Can you work these out from the model? Positions are in its coordinate system, mm. A direction names the side the tool comes from. Coordinates: 2 decimals unless noted, no trailing zeros. Order: outer loops, then holes, each group sorted by start corner. A loop starts at its lowest first (then second) coordinate and runs counter-clockwise, first axis right, second up. Notation, with made-up numbers: (77.5, 77) -> (110.5, 77) arc R19 cw to (110.5, 112) -> close; hole circle Ø1 at (-10, 49.25). An arc over 180 degrees is marked (long way). Answer in a Markdown table with one row per item.
```python
from build123d import *

# Parameters (mm, degrees)
SKETCH_W           = 42
SKETCH_H           = 42
PAD_DEPTH          = 48
CHAMFER_SIZE       = 4
SKETCH001_R        = 11
PAD001_DEPTH       = 2
SKETCH002_R        = 2.5
PAD002_DEPTH       = 24
POCKET_DEPTH       = 15
SKETCH004_R        = 1.25
POCKET001_DEPTH    = 5
POLARPATTERN_COUNT = 4


with BuildPart() as part:
    # Sketch → Pad (new body)
    with BuildSketch(Plane.XY):
        Rectangle(SKETCH_W, SKETCH_H)
    extrude(amount=PAD_DEPTH)

    # Chamfer
    chamfer_edges = [part.edges().sort_by_distance(p)[0] for p in [
        (21, -21, 24),
        (-21, -21, 24),
        (21, 21, 24),
        (-21, 21, 24),
    ]]
    chamfer(chamfer_edges, length=CHAMFER_SIZE)

    # Sketch001 → Pad001 (join)
    with BuildSketch(Plane.XY):
        Circle(SKETCH001_R)
    extrude(amount=-PAD001_DEPTH)

    # Sketch002 (on Face12 of Pad001) → Pad002 (join)
    with BuildSketch(Plane(origin=(0, 0, -2), x_dir=(1, 0, 0), z_dir=(0, 0, -1))):
        Circle(SKETCH002_R)
    extrude(amount=PAD002_DEPTH)

    # Sketch003 (on Face14 of Pad002) → Pocket (cut)
    with BuildSketch(Plane(origin=(0, 0, -26), x_dir=(1, 0, 0), z_dir=(0, 0, -1))):
        with BuildLine():
            ThreePointArc((1.5, 2), (0, 2.5), (-1.5, 2))
            Line((-1.5, 2), (1.5, 2))
        make_face()
    extrude(amount=-POCKET_DEPTH, mode=Mode.SUBTRACT)

    # Sketch004 (on Face2 of Pocket) → Pocket001 (cut)
    with BuildSketch(Plane(origin=(0, 0, 0), x_dir=(1, 0, 0), z_dir=(0, 0, -1))):
        with Locations((15.5, 15.5)):
            Circle(SKETCH004_R)
    pocket001 = extrude(amount=-POCKET001_DEPTH, mode=Mode.SUBTRACT)

    # PolarPattern: Pocket001 ×4 about axis
    polarpattern_axis = Axis((0, 0, 0), (0, 0, 1))
    for i in range(1, POLARPATTERN_COUNT):
        add(pocket001.rotate(polarpattern_axis, i * 360 / POLARPATTERN_COUNT), mode=Mode.SUBTRACT)


solid = part.part
```
(1) I need wall thicknesses on line 1 (Y direction, x = -15.5, z = 2.65); line 2 (Y direction, x = 15, z = 2). Which ranges of each line are inside material? Lowest first, please. Write a range as [from, to].
Response values:
| item | result |
|---|---|
| line 1 | [-21, -16.75], [-14.25, 14.25], [16.75, 21] |
| line 2 | [-21, -16.65], [-14.35, 14.35], [16.65, 21] |
(2) On a 3-axis mill with a long thin cutter (end or side, diameter ignored), from which of +Z, -Z, +X, -X, +Y, -Y can I reach the whole of each face in a straight line? I mean faces 4 (the flat face through (0, -2, -19)), 5 (the cylindrical face through (-14.579, 16.345, 2.465)), 6 (the flat face through (0, 21, 24)). Say none if no direction works.
Response values:
| item | result |
|---|---|
| face 4 | -Z, +X, -X, -Y |
| face 5 | -Z |
| face 6 | +Z, -Z, +X, -X, +Y |
(3) Will these pins go through, and if not, where does the flat tip stop? pin 1 Ø1.5 at (x, y) = (16, -7.5) entering from -Z; pin 2 Ø1.5 at (x, y) = (-15.5, -15.5) entering from -Z; pin 3 Ø0.9 at (x, z) = (0, -20) entering from -Y.
Response values:
| item | result |
|---|---|
| pin 1 | z = 0 |
| pin 2 | z = 5 |
| pin 3 | y = -2 |
(4) Suppose I cut it at C-C (x = 0). Please give me the cut outline in (y, z), and give its area (3 significant figures).
Response values:
| item | result |
|---|---|
| outline | (-21, 0) -> (-11, 0) -> (-11, -2) -> (-2.5, -2) -> (-2.5, -11) -> (-2, -11) -> (-2, -26) -> (2.5, -26) -> (2.5, -2) -> (11, -2) -> (11, 0) -> (21, 0) -> (21, 48) -> (-21, 48) -> close |
| area | 2,170 mm2 |
(5) Suppose I cut it at B-B (z = 28). Please give me the cut outline in (x, y).
Response values:
| item | result |
|---|---|
| outline | (-21, -17) -> (-17, -21) -> (17, -21) -> (21, -17) -> (21, 17) -> (17, 21) -> (-17, 21) -> (-21, 17) -> close |
(6) Suppose I cut it at A-A (y = 0). Please give me the cut outline in (x, z).
Response values:
| item | result |
|---|---|
| outline | (-21, 0) -> (-11, 0) -> (-11, -2) -> (-2.5, -2) -> (-2.5, -26) -> (2.5, -26) -> (2.5, -2) -> (11, -2) -> (11, 0) -> (21, 0) -> (21, 48) -> (-21, 48) -> close |
(7) Suppose I cut it at D-D (y = -15.5). Please give me the cut outline in (x, z), and give its area (3 significant figures).
Response values:
| item | result |
|---|---|
| outline | (-21, 0) -> (-16.75, 0) -> (-16.75, 5) -> (-14.25, 5) -> (-14.25, 0) -> (14.25, 0) -> (14.25, 5) -> (16.75, 5) -> (16.75, 0) -> (21, 0) -> (21, 48) -> (-21, 48) -> close |
| area | 1,990 mm2 |
(8) We'd pull the mould along Y, two halves only. Please class faces 1 (the cylindrical face through (-0.54, 2.44, -13.83)), 2 (the flat face through (-19, -19, 24)), 3 (the flat face through (15, -16, 5)): +Y half, -Y half, draft (parallel to the pull), parting line (faces both ways), or undercut.
Response values:
| item | result |
|---|---|
| face 1 | parting line |
| face 2 | -Y half |
| face 3 | undercut |
